Read the model definition and answer for the solid it produces. Units are mm, in the model's axes. A direction names the side the tool comes from. Round coordinates to 2 decimals unless told otherwise and drop trailing zeros. Write each loop counter-clockwise with the first axis right and the second up, starting at its lowest first coordinate (ties: lowest second). Pieces come first, ordered by that corner, then holes. Notation, with made-up numbers: (8.25, 83) - (63.25, 83) arc R6 cw to (63.25, 90) - close; hole circle Ø10 at (-18.75, -12.75). An arc over 180 degrees is marked (long way). Use one line per item in the form item = value. Start each with the question number.
1) For a pull along Y with two mould halves and no side action, classify faces 1 (the face through (-12.3, 28.8, 42.4)), 2 (the face through (-30.238, 19.016, -42.563)), 3 (the face through (-34.65, 3.01, -0.53)) as released by +Y, released by -Y, zero draft, split by the parting line, or undercut.
2) The part is cut by section A-A, the plane z = -28.5. Give the vertices of the cut face in (x, y).
3) Each of these flat-tipped pins is pushed along its axis until it touches: pin 1 (8 mm diameter, centred on y = 25, z = 30, fed in from +X); pin 2 (1.8 mm diameter, centred on x = 25.5, y = 16, fed in from +Z); pin 3 (4 mm diameter, centred on y = 5, z = -23.5, fed in from -X). Where does it stop, or does it pass through?
4) Consider line 1 along Z through (x, y) = (23.5, 22.5); line 2 along X through (y, z) = (24.5, 13); line 3 along X through (y, z) = (27.75, -32.5). Determine where each line is inside the solid, lowest interval first. Write a range as from..to.
5) The part is cut by section B-B, the plane y = 5.75. Give the vertices of the cut face in (x, z).
6) For faces 4 (the face through (-12.3, 28.8, -42.6)), 5 (the face through (12.3, 28.8, 42.4)), 6 (the face through (-25, 15, 43)), determine the directions among +Z, -Z, +X, -X, +Y, -Y from which every point of the face is accessible in a straight line to the end or side of a thin tool.
from build123d import *

# Parameters (mm, degrees)
SKETCH1_W           = 75
SKETCH1_H           = 94
BOSS_EXTRUDE1_DEPTH = 30
SKETCH2_W           = 20.025762067
SKETCH2_H           = 30
CUT_EXTRUDE5_DEPTH  = 9
SKETCH7_W           = 20.025762067
SKETCH7_H           = 30
CUT_EXTRUDE6_DEPTH  = 9
SKETCH8_R           = 6.6
BOSS_EXTRUDE2_DEPTH = 9
BOSS_EXTRUDE3_START = 9
SKETCH9_R           = 6.6
BOSS_EXTRUDE3_DEPTH = 9
FILLET1_R           = 10
CUT_EXTRUDE7_DEPTH  = 9
CUT_EXTRUDE8_START  = -9
CUT_EXTRUDE8_DEPTH  = 9
FILLET2_R           = 2
CUT_EXTRUDE10_DEPTH = 4
SKETCH14_W          = 37.5
SKETCH14_H          = 30
CUT_EXTRUDE11_DEPTH = 94


with BuildPart() as part:
    # Sketch1 → Boss-Extrude1 (new body)
    with BuildSketch(Plane(origin=(0, 0, 0), x_dir=(1, 0, 0), z_dir=(0, 1, 0))):
        Rectangle(SKETCH1_W, SKETCH1_H)
    extrude(amount=BOSS_EXTRUDE1_DEPTH)

    # Sketch2 → Cut-Extrude5 (cut)
    with BuildSketch(Plane.XY.offset(47)):
        with Locations((-27.487118966, 15)):
            Rectangle(SKETCH2_W, SKETCH2_H)
    extrude(amount=-CUT_EXTRUDE5_DEPTH, mode=Mode.SUBTRACT)

    # Sketch7 → Cut-Extrude6 (cut)
    with BuildSketch(Plane(origin=(0, 0, -47), x_dir=(-1, 0, 0), z_dir=(0, 0, -1))):
        with Locations((27.487118966, 15)):
            Rectangle(SKETCH7_W, SKETCH7_H)
    extrude(amount=-CUT_EXTRUDE6_DEPTH, mode=Mode.SUBTRACT)

    # Sketch8 → Boss-Extrude2 (add)
    with BuildSketch(Plane.XY.offset(38)):
        with Locations((-25, 15)):
            Circle(SKETCH8_R)
    extrude(amount=BOSS_EXTRUDE2_DEPTH)

    # Sketch9 → Boss-Extrude3 (add)
    with BuildSketch(Plane(origin=(0, 0, -38), x_dir=(-1, 0, 0), z_dir=(0, 0, -1)).offset(BOSS_EXTRUDE3_START)):
        with Locations(Location((25, 15, 0), (0, 0, 180))):
            Circle(SKETCH9_R)
    extrude(amount=-BOSS_EXTRUDE3_DEPTH)

    # Fillet1
    fillet1_edges = [part.edges().sort_by_distance(p)[0] for p in [
        (-37.5, 0, 0),
        (-37.5, 30, 0),
    ]]
    fillet(fillet1_edges, radius=FILLET1_R)

    # Sketch10 → Cut-Extrude7 (cut)
    with BuildSketch(Plane.XY.offset(47)):
        with BuildLine():
            Line((-15.986121811, 30), (-17.474237933, 30))
            Line((-17.474237933, 30), (-17.474237933, 0))
            Line((-17.474237933, 0), (-15.986121811, 0))
            ThreePointArc((-15.986121811, 0), (-7.5, 15), (-15.986121811, 30))
        make_face()
    extrude(amount=-CUT_EXTRUDE7_DEPTH, mode=Mode.SUBTRACT)

    # Sketch11 → Cut-Extrude8 (cut)
    with BuildSketch(Plane(origin=(0, 0, -47), x_dir=(-1, 0, 0), z_dir=(0, 0, -1)).offset(CUT_EXTRUDE8_START)):
        with BuildLine():
            Line((15.986121811, 30), (17.474237933, 30))
            Line((17.474237933, 30), (17.474237933, 0))
            Line((17.474237933, 0), (15.986121811, 0))
            ThreePointArc((15.986121811, 0), (7.5, 15), (15.986121811, 30))
        make_face()
    extrude(amount=CUT_EXTRUDE8_DEPTH, mode=Mode.SUBTRACT)

    # Fillet2
    fillet2_edges = [part.edges().sort_by_distance(p)[0] for p in [
        (-15.986121811, 30, 42.5),
        (-15.986121811, 0, 42.5),
        (-15.986121811, 0, -42.5),
        (-15.986121811, 30, -42.5),
    ]]
    fillet(fillet2_edges, radius=FILLET2_R)

    # Sketch13 → Cut-Extrude10 (cut)
    with BuildSketch(Plane.XY.offset(47)):
        Polygon((-26.622500709, 17.20554754), (-26.458244341, 17.605297016), (-26.032711731, 17.529786775), (-25.774202126, 17.876128488), (-25.380817039, 17.697164883), (-25.044297307, 17.96833691), (-24.707777575, 17.697164883), (-24.314392488, 17.876128488), (-24.055882883, 17.529786775), (-23.630350274, 17.605297016), (-23.466093905, 17.20554754), (-23.035151551, 17.172859831), (-22.97546925, 16.744820322), (-22.566194846, 16.605988553), (-22.614836671, 16.176554308), (-22.252946432, 15.940301788), (-22.406856039, 15.53645574), (-22.115088859, 15.217627085), (-22.364595541, 14.864744365), (-22.161284226, 14.483372752), (-22.490710561, 14.20362628), (-22.388629908, 13.783674689), (-22.777276827, 13.594641965), (-22.782840939, 13.1624975), (-23.206288328, 13.076056145), (-23.319147592, 12.658872031), (-23.750788692, 12.680453474), (-23.963851745, 12.304442924), (-24.37656496, 12.432691122), (-24.676444267, 12.121480262), (-25.044297307, 12.34833691), (-25.412150348, 12.121480262), (-25.712029654, 12.432691122), (-26.124742869, 12.304442924), (-26.337805922, 12.680453474), (-26.769447023, 12.658872031), (-26.882306286, 13.076056145), (-27.305753675, 13.1624975), (-27.311317787, 13.594641965), (-27.699964706, 13.783674689), (-27.597884053, 14.20362628), (-27.927310388, 14.483372752), (-27.723999073, 14.864744365), (-27.973505755, 15.217627085), (-27.681738575, 15.53645574), (-27.835648182, 15.940301788), (-27.473757943, 16.176554308), (-27.522399768, 16.605988553), (-27.113125364, 16.744820322), (-27.053443063, 17.172859831), align=None)
    extrude(amount=-CUT_EXTRUDE10_DEPTH, mode=Mode.SUBTRACT)

    # Sketch14 → Cut-Extrude11 (cut)
    with BuildSketch(Plane.XY.offset(47)):
        with Locations((18.75, 15)):
            Rectangle(SKETCH14_W, SKETCH14_H)
    extrude(amount=-CUT_EXTRUDE11_DEPTH, mode=Mode.SUBTRACT)

    # Mirror2: part across plane


with BuildPart() as part_1:
    add(part.part)
    add(part.part.mirror(Plane(origin=(0, 0, -47), x_dir=(0, 0, 1), z_dir=(-1, 0, 0))))


solid = part_1.part
Geometry results:
q1.face_1 = undercut
q1.face_2 = split by the parting line
q1.face_3 = released by -Y
q2.outline = (-37.5, 10) arc R10 ccw to (-27.5, 0) - (27.5, 0) arc R10 ccw to (37.5, 10) - (37.5, 20) arc R10 ccw to (27.5, 30) - (-27.5, 30) arc R10 ccw to (-37.5, 20) - close
q3.pin_1 = 37.45
q3.pin_2 = 43
q3.pin_3 = -37.04
q4.line_1 = -38..38
q4.line_2 = -36.43..36.43
q4.line_3 = -33.82..33.82
q5.outline = (-36.55, -38) - (-10.14, -38) - (-10.14, -47) - (10.14, -47) - (10.14, -38) - (36.55, -38) - (36.55, 38) - (10.14, 38) - (10.14, 47) - (-10.14, 47) - (-10.14, 38) - (-36.55, 38) - close
q6.face_4 = -Z, -X
q6.face_5 = +Z, +X
q6.face_6 = +Z
